from build123d import *

# Parameters (mm, degrees)
BASE_FLANGE1_DEPTH = 63.5
HOLE1_START        = 28.172610526
HOLE1_OUTLINE_R    = 1.5
HOLE1_DEPTH        = 0.7366
SKETCH8_W          = 6.35
SKETCH8_H          = 6.35
CUT_EXTRUDE1_DEPTH = 90.436486872


# Read off the part's stored shape, not the designer's step: Hole1
# Sheet-metal steps are written as plain solids
with BuildPart() as part:
    # Sketch2 → Base-Flange1 (new body)
    with BuildSketch(Plane(origin=(0, 0, 0), x_dir=(0, 0, -1), z_dir=(1, 0, 0))):
        with BuildLine():
            Line((-28.909210526, -21.807236842), (-28.909210526, -10.580436842))
            ThreePointArc((-28.909210526, -10.580436842), (-28.477720236, -9.538727132), (-27.436010526, -9.107236842))
            Line((-27.436010526, -9.107236842), (2.104189474, -9.107236842))
            ThreePointArc((2.104189474, -9.107236842), (2.625044329, -8.891491697), (2.840789474, -8.370636842))
            Line((2.840789474, -8.370636842), (2.840789474, 54.392763158))
            Line((2.840789474, 54.392763158), (3.577389474, 54.392763158))
            Line((3.577389474, 54.392763158), (3.577389474, -8.370636842))
            ThreePointArc((3.577389474, -8.370636842), (3.145899184, -9.412346552), (2.104189474, -9.843836842))
            Line((2.104189474, -9.843836842), (-27.436010526, -9.843836842))
            ThreePointArc((-27.436010526, -9.843836842), (-27.956865381, -10.059581987), (-28.172610526, -10.580436842))
            Line((-28.172610526, -10.580436842), (-28.172610526, -21.807236842))
            Line((-28.172610526, -21.807236842), (-28.909210526, -21.807236842))
        make_face()
    extrude(amount=BASE_FLANGE1_DEPTH)

    # Hole1 outline → Hole1 (cut)
    with BuildSketch(Plane.XY.offset(HOLE1_START)):
        with Locations((6.35, -19.368836842)):
            Circle(HOLE1_OUTLINE_R)
        with Locations((57.15, -19.368836842)):
            Circle(HOLE1_OUTLINE_R)
    extrude(amount=HOLE1_DEPTH, mode=Mode.SUBTRACT)

    # Sketch8 → Cut-Extrude1 (cut, through all)
    with BuildSketch(Plane.XY.offset(-2.840789474)):
        with Locations((31.75, 32.167763158)):
            Rectangle(SKETCH8_W, SKETCH8_H)
    extrude(amount=-CUT_EXTRUDE1_DEPTH, mode=Mode.SUBTRACT)


solid = part.part
Can you work these out from the model? Positions are in its coordinate system, mm. A direction names the side the tool comes from. Give positions to 0.01 mm unless a question says otherwise; leave off trailing zeros. Write each loop counter-clockwise with the first axis right and the second up, starting at its lowest first coordinate (ties: lowest second). Pieces come first, ordered by that corner, then holes. Notation, with made-up numbers: M 50,-21 L 79,-21 A25 cw 79,6 Z; hole C 65.5,1 d6. An arc over 180 degrees is marked long. Answer in a Markdown table with one row per item. Add a question column.
Item 1: Imagine slicing it at D-D, the plane z = 9. Write out the boundary of the cut face in (x, y), plus the area to 3 significant figures.
Item 2: On a 3-axis mill with a long thin cutter (end or side, diameter ignored), from which of +Z, -Z, +X, -X, +Y, -Y can I reach the whole of each face in a straight line? I mean faces 4 (the flat face through (0, 16, -3)), 5 (the flat face through (31, 23, -2.841)), 6 (the flat face through (31, -9.844, 12)). Say none if no direction works.
Item 3: Imagine slicing it at C-C, the plane y = 15. Write out the boundary of the cut face in (x, z).
Item 4: We'd pull the mould along X, two halves only. Please class faces 1 (the flat face through (31, -9.107, 13)), 2 (the cylindrical face through (56.825, -20.833, 28.536)), 3 (the flat face through (63.5, 16, -3)): released by +X, released by -X, zero draft, split by the parting line, or undercut.
Item 5: Imagine slicing it at A-A, the plane x = 6.35. Write out the boundary of the cut face in (y, z).
Item 6: Please list where these lines run through material, in increasing order: L1, parallel to Z at x = 35.5, y = 38; L2, parallel to Y at x = 41, z = 14; L3, parallel to Y at x = 57.15, z = 28.7.
Item 7: Imagine slicing it at B-B, the plane x = 26. Write out the boundary of the cut face in (y, z), plus the area to 3 significant figures.
Item 8: For pin 1 Ø9 at (x, y) = (24, -17.5) entering from -Z; pin 2 Ø10 at (x, z) = (51.5, 16) entering from +Y; pin 3 Ø0.6 at (x, z) = (31.5, -3) entering from -Y, each with a flat end and sliding along its axis, tell me the tip position at first contact or that it passes through.
Evaluation:
| question | item | result |
|---|---|---|
| 1 | outline | M 0,-9.84 L 63.5,-9.84 L 63.5,-9.11 L 0,-9.11 Z |
| 1 | area | 46.8 mm² |
| 2 | face 4 | +Z, -Z, -X, +Y, -Y |
| 2 | face 5 | +Z, +X, -X, +Y |
| 2 | face 6 | -Z, +X, -X, -Y |
| 3 | outline | M 0,-3.58 L 63.5,-3.58 L 63.5,-2.84 L 0,-2.84 Z |
| 4 | face 1 | zero draft |
| 4 | face 2 | undercut |
| 4 | face 3 | released by +X |
| 5 | outline | M -21.81,28.17 L -20.87,28.17 L -20.87,28.91 L -21.81,28.91 Z; M -17.87,28.17 L -10.58,28.17 A0.74 cw -9.84,27.44 L -9.84,-2.1 A1.47 ccw -8.37,-3.58 L 54.39,-3.58 L 54.39,-2.84 L -8.37,-2.84 A0.74 cw -9.11,-2.1 L -9.11,27.44 A1.47 ccw -10.58,28.91 L -17.87,28.91 Z |
| 6 | L1 | z = -3.58 to -2.84 |
| 6 | L2 | y = -9.84 to -9.11 |
| 6 | L3 | y = -21.81 to -20.87, -17.87 to -9.82 |
| 7 | outline | M -21.81,28.17 L -10.58,28.17 A0.74 cw -9.84,27.44 L -9.84,-2.1 A1.47 ccw -8.37,-3.58 L 54.39,-3.58 L 54.39,-2.84 L -8.37,-2.84 A0.74 cw -9.11,-2.1 L -9.11,27.44 A1.47 ccw -10.58,28.91 L -21.81,28.91 Z |
| 7 | area | 78.8 mm² |
| 8 | pin 1 | stops at z = 28.17 |
| 8 | pin 2 | stops at y = -9.11 |
| 8 | pin 3 | stops at y = -9.72 |
